Verification items for the finished model (mm, model axes). Face numbers are marked on the shaded views. A direction names the side the tool comes from. Coordinates: 2 decimals unless noted, no trailing zeros. Loops run counter-clockwise (first coordinate to the right, second up) from the corner with the lowest first, then second, coordinate; pieces in that order, holes last. Notation, with made-up numbers: (38.5, 17.5) -> (64.5, 17.5) arc R31 cw to (64.5, 42.5) -> close; hole circle Ø8 at (-28.5, 36). An arc over 180 degrees is marked (long way). Write item = value, one per line.
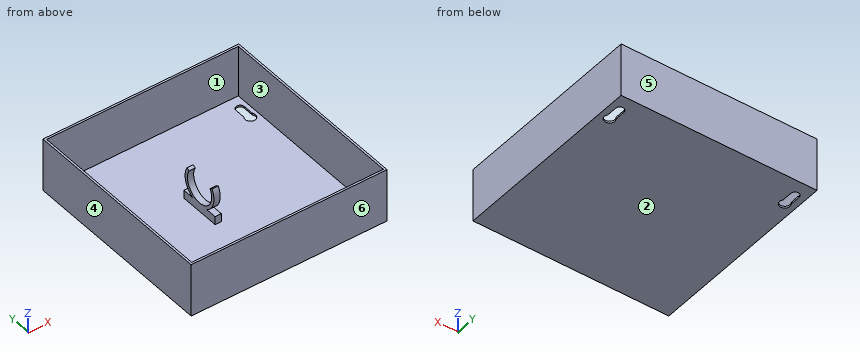
```python
from build123d import *

# Parameters (mm, degrees)
CROQUIS1_W              = 95
CROQUIS1_H              = 95
SALIENTE_EXTRUIR1_DEPTH = 0.9
CROQUIS2_W              = 95
CROQUIS2_H              = 95
CROQUIS2_W_2            = 93
CROQUIS2_H_2            = 93
SALIENTE_EXTRUIR2_DEPTH = 25
CROQUIS3_W              = 3
CROQUIS3_H              = 20
SALIENTE_EXTRUIR3_DEPTH = 4
SALIENTE_EXTRUIR4_START = -3
SALIENTE_EXTRUIR4_DEPTH = 3


with BuildPart() as part:
    # Croquis1 → Saliente-Extruir1 (new body)
    with BuildSketch(Plane.XY):
        Rectangle(CROQUIS1_W, CROQUIS1_H)
        with BuildLine():
            Line((-44.5, 39.976525822), (-44.5, 34.976525822))
            ThreePointArc((-44.5, 34.976525822), (-42.5, 30.976525822), (-40.5, 34.976525822))
            Line((-40.5, 34.976525822), (-40.5, 39.976525822))
            ThreePointArc((-40.5, 39.976525822), (-42.5, 41.976525822), (-44.5, 39.976525822))
        make_face(mode=Mode.SUBTRACT)
        with BuildLine():
            Line((40.5, 39.976525822), (40.5, 34.976525822))
            ThreePointArc((40.5, 34.976525822), (42.5, 30.976525822), (44.5, 34.976525822))
            Line((44.5, 34.976525822), (44.5, 39.976525822))
            ThreePointArc((44.5, 39.976525822), (42.5, 41.976525822), (40.5, 39.976525822))
        make_face(mode=Mode.SUBTRACT)
    extrude(amount=SALIENTE_EXTRUIR1_DEPTH)

    # Croquis2 → Saliente-Extruir2 (add)
    with BuildSketch(Plane.XY.offset(0.9)):
        Rectangle(CROQUIS2_W, CROQUIS2_H)
        Rectangle(CROQUIS2_W_2, CROQUIS2_H_2, mode=Mode.SUBTRACT)
    extrude(amount=SALIENTE_EXTRUIR2_DEPTH)

    # Croquis3 → Saliente-Extruir3 (add)
    with BuildSketch(Plane.XY.offset(0.9)):
        with Locations((-6, 0)):
            Rectangle(CROQUIS3_W, CROQUIS3_H)
    extrude(amount=SALIENTE_EXTRUIR3_DEPTH)

    # Croquis4 → Saliente-Extruir4 (add)
    with BuildSketch(Plane.ZY.offset(7.5).offset(SALIENTE_EXTRUIR4_START)):
        with BuildLine():
            Line((17.575, 8.010734985), (16.825, 6.711696879))
            ThreePointArc((16.825, 6.711696879), (5.2, 0), (16.825, -6.711696879))
            Line((16.825, -6.711696879), (17.575, -8.010734985))
            ThreePointArc((17.575, -8.010734985), (10.517735249, -8.924493721), (4.9, -4.5563143))
            Line((4.9, -4.5563143), (4.9, 4.5563143))
            ThreePointArc((4.9, 4.5563143), (10.517735249, 8.924493721), (17.575, 8.010734985))
        make_face()
    extrude(amount=SALIENTE_EXTRUIR4_DEPTH)


solid = part.part
```
1) Depth check by flat-ended pin: pin 1 Ø1.5 at (x, y) = (3, -34) entering from +Z; pin 2 Ø3.5 at (x, y) = (-6, -6.5) entering from +Z (3 decimals); pin 3 Ø3.5 at (x, y) = (-6.5, 6) entering from +Z. Enter the tip coordinate at first touch or a pass-through.
Ans:
pin_1 = 0.9
pin_2 = 17.575
pin_3 = 17.42
2) Material ranges on line 1 (X direction, y = 40, z = 15.25); line 2 (Y direction, x = 42.5, z = 0.65), recorded low to high.
Ans:
line_1 = -47.5 to -46.5, 46.5 to 47.5
line_2 = -47.5 to 30.98, 41.98 to 47.5
3) Tool access check on the marked faces 1 and 2. Record the directions out of +Z, -Z, +X, -X, +Y, -Y that give a thin tool (end or side, any length) a straight path to the whole face; none if there is none.
Ans:
face_1 = +Z
face_2 = -Z, +X, -X, +Y, -Y
4) Sectioned sample at C-C, the plane y = 0. Record the cut outline in (x, z).
Ans:
outline = (-47.5, 0) -> (47.5, 0) -> (47.5, 25.9) -> (46.5, 25.9) -> (46.5, 0.9) -> (-4.5, 0.9) -> (-4.5, 5.2) -> (-7.5, 5.2) -> (-7.5, 0.9) -> (-46.5, 0.9) -> (-46.5, 25.9) -> (-47.5, 25.9) -> close
5) Sectioned sample at B-B, the plane x = -42.5. Record the cut outline in (y, z).
Ans:
outline = (-47.5, 0) -> (30.98, 0) -> (30.98, 0.9) -> (-46.5, 0.9) -> (-46.5, 25.9) -> (-47.5, 25.9) -> close; (41.98, 0) -> (47.5, 0) -> (47.5, 25.9) -> (46.5, 25.9) -> (46.5, 0.9) -> (41.98, 0.9) -> close
6) Sectioned sample at A-A, the plane z = 12.95. Record the cut outline in (x, y), plus the area to 3 significant figures.
Ans:
outline = (-47.5, -47.5) -> (47.5, -47.5) -> (47.5, 47.5) -> (-47.5, 47.5) -> close; (-7.5, -9.25) -> (-4.5, -9.25) -> (-4.5, -7.75) -> (-7.5, -7.75) -> close; (-7.5, 7.75) -> (-4.5, 7.75) -> (-4.5, 9.25) -> (-7.5, 9.25) -> close; hole (-46.5, -46.5) -> (46.5, -46.5) -> (46.5, 46.5) -> (-46.5, 46.5) -> close
area = 385 mm2
7) Sectioned sample at D-D, the plane z = 22.5. Record the cut outline in (x, y), plus the area to 3 significant figures.
Ans:
outline = (-47.5, -47.5) -> (47.5, -47.5) -> (47.5, 47.5) -> (-47.5, 47.5) -> close; hole (-46.5, -46.5) -> (46.5, -46.5) -> (46.5, 46.5) -> (-46.5, 46.5) -> close
area = 376 mm2
8) Release check for a two-part mould opening along Y. For the marked faces 3, 4, 5 and 6 record: pulls with the +Y half, pulls with the -Y half, needs draft (parallel to the pull), parting line crosses it, or undercut.
Ans:
face_3 = undercut
face_4 = needs draft
face_5 = pulls with the +Y half
face_6 = pulls with the -Y half
